Source: CAD feature listing. Evaluate the final solid. Frame: model axes, mm. A direction names the side the tool comes from. Give positions to 0.01 mm unless a question says otherwise; leave off trailing zeros. Order: outer loops, then holes, each group sorted by start corner. A loop starts at its lowest first (then second) coordinate and runs counter-clockwise, first axis right, second up. Notation, with made-up numbers: M 14.25,-4 L 66.25,-4 A9 cw 66.25,7 Z; hole C 30.5,-1.75 d3. An arc over 180 degrees is marked long. Answer in a Markdown table with one row per item. Add a question column.
(1) Section query D-D, the plane y = 25. Return loops of the section in (x, z), plus the area to 3 significant figures.
(2) Pin query (flat end, axial travel): P1, Ø5, axis at y = -6, z = -16, coming from the -X side; P2, Ø1, axis at x = -8, z = 19, coming from the -Y side; P3, Ø8, axis at x = -10, y = -10.5, coming from the -Z side. Return the tip coordinate at first contact, or that it passes through.
(3) Section query C-C, the plane z = 20. Return loops of the section in (x, y).
(4) Section query B-B, the plane x = -21. Return loops of the section in (y, z), plus the area to 3 significant figures.
(5) Material intervals for line 1 along Z through (x, y) = (0, -4); line 2 along Y through (x, z) = (-5, -4.5); line 3 along Y through (x, z) = (-20, -11), sorted ascending.
(6) Section query A-A, the plane x = 0. Return loops of the section in (y, z).
(7) Set-up query: faces 1 (the face through (-17.52, -5.07, 0.78)), 2 (the face through (1.08, 29.58, -4.88)), 3 (the face through (13, -10, 0)). Return all of +Z, -Z, +X, -X, +Y, -Y with unobstructed straight access to the full face (end or side cutting, diameter ignored); none if empty.
from build123d import *

# Parameters (mm, degrees)
F0_R     = 30
F1_DEPTH = 10
F2_R     = 2.6
F3_DEPTH = 25
F4_R     = 10
F5_DEPTH = 10
F6_R     = 5
F7_DEPTH = 60


with BuildPart() as f1:
    # F0 (on Front) → F1 (new body)
    with BuildSketch(Plane.XZ):
        Circle(F0_R)
    extrude(amount=F1_DEPTH)

    # F2 (on face) → F3 (cut)
    with BuildSketch(Plane.XZ.offset(10)):
        with Locations((-20, 0)):
            Circle(F2_R)
        with Locations((0, 20)):
            Circle(F2_R)
        with Locations((20, 0)):
            Circle(F2_R)
        with Locations((0, -20)):
            Circle(F2_R)
    extrude(amount=-F3_DEPTH, mode=Mode.SUBTRACT)

    # F4 (on face) → F5 (join)
    with BuildSketch(Plane.XZ.offset(10)):
        Circle(F4_R)
    extrude(amount=F5_DEPTH)

    # F6 (on face) → F7 (join)
    with BuildSketch(Plane(origin=(0, 0, 0), x_dir=(-1, 0, 0), z_dir=(0, 1, 0))):
        Circle(F6_R)
    extrude(amount=F7_DEPTH)


solid = f1.part
Values follow:
| question | item | result |
|---|---|---|
| 1 | outline | C 0,0 d10 |
| 1 | area | 78.5 mm² |
| 2 | P1 | stops at x = -26.79 |
| 2 | P2 | stops at y = -10 |
| 2 | P3 | stops at z = -29.39 |
| 3 | outline | M -22.36,-10 L -2.6,-10 L -2.6,0 L -22.36,0 Z; M 2.6,-10 L 22.36,-10 L 22.36,0 L 2.6,0 Z |
| 4 | outline | M -10,-21.42 L 0,-21.42 L 0,-2.4 L -10,-2.4 Z; M -10,2.4 L 0,2.4 L 0,21.42 L -10,21.42 Z |
| 4 | area | 380 mm² |
| 5 | line 1 | z = -30 to -22.6, -17.4 to 17.4, 22.6 to 30 |
| 5 | line 2 | y = -20 to 0 |
| 5 | line 3 | y = -10 to 0 |
| 6 | outline | M -20,-10 L -10,-10 L -10,-17.4 L 0,-17.4 L 0,-5 L 60,-5 L 60,5 L 0,5 L 0,17.4 L -10,17.4 L -10,10 L -20,10 Z; M -10,-30 L 0,-30 L 0,-22.6 L -10,-22.6 Z; M -10,22.6 L 0,22.6 L 0,30 L -10,30 Z |
| 7 | face 1 | +Y, -Y |
| 7 | face 2 | +Y |
| 7 | face 3 | -Y |
